Autodesk Inventor part; units mm, degrees
ref_plane "YZ Plane" through (0, 0, 0) normal (1, 0, 0) x (0, 1, 0)
ref_plane "XZ Plane" through (0, 0, 0) normal (0, 1, 0) x (-1, 0, 0)
ref_plane "XY Plane" through (0, 0, 0) normal (0, 0, 1) x (1, 0, 0)
sketch "Szkic7" plane through (0, 0, 0) normal (0, 0, 1) x (1, 0, 0)
  circle A0 centre (0, 0) radius 37.592
  dimension "d35" = 75.184
extrude "Wyciągnięcie proste2" add sketch "Szkic7" along normal mid plane 32.45
chamfer "Faza2" distance 1 angle 45 1 edges at (-37.592, 0, 16.225)
sketch "Szkic9" plane through (0, 0, 16.225) normal (0, 0, 1) x (1, 0, 0)
  circle A0 centre (0, 0) radius 36.592
extrude "Wyciągnięcie proste3" add sketch "Szkic9" along normal blind 2.75
sketch "Szkic10" plane through (0, 0, 18.975) normal (0, 0, 1) x (1, 0, 0)
  line L0 (-23.3827, 40.5) -> (23.3827, 40.5)
  line L1 (23.3827, 40.5) -> (46.7654, 0)
  line L2 (46.7654, 0) -> (23.3827, -40.5)
  line L3 (23.3827, -40.5) -> (-23.3827, -40.5)
  line L4 (-23.3827, -40.5) -> (-46.7654, 0)
  line L5 (-46.7654, 0) -> (-23.3827, 40.5)
  line L6 (0, 52.6288) -> (0, -52.6288) construction
  line L7 (-52.6288, 0) -> (52.6288, 0) construction
  point P0 (0, 0)
  point P1 (0, 0)
  point P2 (0, 40.5)
  dimension "d44" = 81
extrude "Wyciągnięcie proste4" add sketch "Szkic10" along normal blind 8.8
sketch "Szkic12" plane through (0, 0, 0) normal (0, 1, 0) x (-1, 0, 0)
  line L0 (0, -2.1463) -> (0, 12.8775) construction
  line L1 (-23.3827, 18.975) -> (-23.3827, 27.775) construction
  line L2 (-46.7654, 27.775) -> (-23.3827, 27.775) construction
  line L3 (-46.7654, 18.975) -> (-46.7654, 27.775)
  line L4 (-46.7654, 26.3281) -> (-41.3654, 27.775)
  line L5 (-46.7654, 27.775) -> (-23.3827, 27.775)
  line L6 (-46.7654, 18.975) -> (-23.3827, 18.975)
  point P0 (0, 0)
  dimension "d50" = 15
  dimension "d51" = 5.4
revolve "Obrót2" cut sketch "Szkic12" angle 360 about axis through (0, 0, -10) along (0, 0, 1)
thread "Gwint3"
chamfer "Faza3" distance 1 angle 45 1 edges at (-37.592, 0, -16.225)
equation "\"d35\" = OD"
equation "\"d36\" = 0.7375 * L"
equation "\"d42\" = 0.0625 * L"
equation "\"d44\" = SW"
equation "\"d45\" = 0.2 * L"
equation "\"d51\" = 0.0666667 * SW"
equation "\"SzerokośćGięciaPodcięcia\" = Grubość"
equation "\"RozmiarPodcięciaNarożnika\" = 4 * Grubość"
equation "\"PromieńPrzejścia\" = PromieńGięcia"
equation "\"Rozmiar_promienia_Jacobiego\" = PromieńGięcia"
equation "\"Wielk_odstępu\" = Grubość"
equation "\"d2\" = PromieńGięcia"
equation "\"d23\" = PromieńGięcia"
equation "\"OD\" = 75.184"
equation "\"SW\" = 81"
equation "\"L\" = 44"
properties part number "Korek sześciokątny BSP 2 1/2'' L=44" material "304"
Verification items for the finished model (mm, model axes). A direction names the side the tool comes from. Round coordinates to 2 decimals unless told otherwise and drop trailing zeros. Write each loop counter-clockwise with the first axis right and the second up, starting at its lowest first coordinate (ties: lowest second). Pieces come first, ordered by that corner, then holes. Notation, with made-up numbers: (37, 24) - (91, 24) arc R13 cw to (91, 36) - close; hole circle Ø1 at (-20.5, 70). An arc over 180 degrees is marked (long way). Answer as a JSON object with one key per item and string values. Group by question number.
Q1. Go/stop test with flat-tipped pins: pin 1 Ø6 at (x, z) = (3.5, 9) entering from +Y; pin 2 Ø10 at (x, z) = (-8, -10) entering from -Y; pin 3 Ø10 at (x, z) = (-29.5, -1.5) entering from -Y. Record where each tip stops, or that it passes through.
Q2. Section check A-A, the plane x = 0. Enter the section's corners in (y, z) (3 decimals), plus the area to 3 significant figures.
Q3. Tool access check on faces 5 (the conical face through (-42.903, -0.191, 27.363)), 6 (the cylindrical face through (-4.894, 37.272, 0.213)), 7 (the flat face through (17, 33, 18.975)). Record the directions out of +Z, -Z, +X, -X, +Y, -Y that give a thin tool (end or side, any length) a straight path to the whole face; none if there is none.
Q4. Section check B-B, the plane z = 11. Enter the section's corners in (x, y).
Q5. Mould release check, pull along Z, two halves, no side actions. Record for faces 1 (the cylindrical face through (34.9, -11, 17.6)), 2 (the flat face through (-1, 1, 27.775)), 3 (the flat face through (-34.91, -20.534, 23.313)), 4 (the flat face through (-1, 1, -16.225)): released by +Z, released by -Z, zero draft, split by the parting line, or undercut.
Q6. Thickness scan on line 1 (Z direction, x = -11.5, y = -36) (3 decimals); line 2 (X direction, y = -8.5, z = -12); line 3 (X direction, y = -23, z = 16). Record the ranges inside material, lowest first.
Found:
{
 "1": {"pin 1": "stops at y = 37.59", "pin 2": "stops at y = -37.47", "pin 3": "stops at y = -28.51"},
 "2": {"outline": "(-40.5, 18.975) - (-36.592, 18.975) - (-36.592, 16.225) - (-37.592, 15.225) - (-37.592, -15.225) - (-36.592, -16.225) - (36.592, -16.225) - (37.592, -15.225) - (37.592, 15.225) - (36.592, 16.225) - (36.592, 18.975) - (40.5, 18.975) - (40.5, 27.775) - (-40.5, 27.775) - close", "area": "3,350 mm^2"},
 "3": {"face 5": "+Z, -X", "face 6": "-Z", "face 7": "none"},
 "4": {"outline": "circle Ø75.18 at (0, 0)"},
 "5": {"face 1": "undercut", "face 2": "released by +Z", "face 3": "zero draft", "face 4": "released by -Z"},
 "6": {"line 1": "z = 18.975 to 27.775", "line 2": "x = -36.62 to 36.62", "line 3": "x = -28.75 to 28.75"}
}
